```python
from build123d import *

# Parameters (mm, degrees)
SKETCH_1_R      = 20
SKETCH_1_R_2    = 1.55
EXTRUDE_1_DEPTH = 3


with BuildPart() as part:
    # 草图1 → 凸台-拉伸1 (new body)
    with BuildSketch(Plane.XY):
        with BuildLine():
            Line((-4, 6), (-4, 0))
            ThreePointArc((-4, 0), (-7.907990216, -19.039432765), (-19, -35))
            ThreePointArc((-19, -35), (-39.34333678, -74.530954843), (4.648648649, -68.108108108))
            ThreePointArc((4.648648649, -68.108108108), (13.142724005, -34.523787334), (16, 0))
            ThreePointArc((16, 0), (15.97856596, 3.000306232), (15.914268214, 6))
            Line((15.914268214, 6), (-4, 6))
        make_face()
        with Locations((-19, -60)):
            Circle(SKETCH_1_R, mode=Mode.SUBTRACT)
        with BuildLine():
            ThreePointArc((-10.997130101, -35.262294501), (-2.27235419, -21.118936487), (1.769449507, -5))
            Line((1.769449507, -5), (9.938716285, -5))
            ThreePointArc((9.938716285, -5), (8.233133382, -26.791038845), (4.205881516, -48.274512246))
            ThreePointArc((4.205881516, -48.274512246), (-2.093610856, -40.247177262), (-10.997130101, -35.262294501))
        make_face(mode=Mode.SUBTRACT)
        Circle(SKETCH_1_R_2, mode=Mode.SUBTRACT)
        with Locations((12, 0)):
            Circle(SKETCH_1_R_2, mode=Mode.SUBTRACT)
    extrude(amount=EXTRUDE_1_DEPTH)


solid = part.part
```
Verification items for the finished model (mm, model axes). A direction names the side the tool comes from. Round coordinates to 2 decimals unless told otherwise and drop trailing zeros. Write each loop counter-clockwise with the first axis right and the second up, starting at its lowest first coordinate (ties: lowest second). Pieces come first, ordered by that corner, then holes.
1. Gauge pin test, flat end, axial feed: P1, Ø1, axis at x = -14, z = 2.5, coming from the -Y side. Record the tip position at first contact, or that the pin passes through.
2. Access from +Z, -Z, +X, -X, +Y, -Y to the whole of each face (thin tool, end or side, straight path). Record for faces 1 (the flat face through (-5, -39, 3)), 2 (the flat face through (-4, 3, 1)), 3 (the flat face through (6, -5, 1)).
3. Draft check along X on faces 4 (the cylindrical face through (0.715, -1.375, 1.479)), 5 (the flat face through (-5, -39, 0)), 6 (the cylindrical face through (-7.8, -18.79, 1.48)). Enter one of: +X half, -X half, draft (parallel to the pull), parting line (faces both ways), or undercut.
4. Section check C-C on x = 0. Enter the section's corners in (y, z) (3 decimals), plus the area to 3 significant figures.
5. Section check A-A on z = 1.05. Enter the section's corners in (x, y).
6. Section check D-D on y = -28. Enter the section's corners in (x, z).
7. Scan lines: L1, parallel to Y at x = -3.5, z = 2.65; L2, parallel to X at y = -0.5, z = 2.2; L3, parallel to Y at x = -19, z = 1.5. Record each from-to range of solid material in increasing order.
8. Section check B-B on y = -43. Enter the section's corners in (x, z).
Answer:
1. P1: stops at y = -84.59
2. face 1: +Z, +X, -X, +Y, -Y
2. face 2: +Z, -Z, -X, +Y
2. face 3: +Z, -Z
3. face 4: undercut
3. face 5: draft
3. face 6: -X half
4. outline: (-76.248, 0) - (-66.245, 0) - (-66.245, 3) - (-76.248, 3) - close; (-53.755, 0) - (-42.252, 0) - (-42.252, 3) - (-53.755, 3) - close; (-14.606, 0) - (-1.55, 0) - (-1.55, 3) - (-14.606, 3) - close; (1.55, 0) - (6, 0) - (6, 3) - (1.55, 3) - close
4. area: 117 mm2
5. outline: (-19, -35) arc R25 ccw (long way) to (4.65, -68.11) arc R210 ccw to (16, 0) arc R210 ccw to (15.91, 6) - (-4, 6) - (-4, 0) arc R48.33 cw to start; hole circle Ø40 at (-19, -60); hole (-11, -35.26) arc R26 cw to (4.21, -48.27) arc R204 ccw to (9.94, -5) - (1.77, -5) arc R54.33 cw to start; hole circle Ø3.1 at (0, 0); hole circle Ø3.1 at (12, 0)
6. outline: (-12.94, 0) - (-5.77, 0) - (-5.77, 3) - (-12.94, 3) - close; (8.07, 0) - (14.12, 0) - (14.12, 3) - (8.07, 3) - close
7. L1: y = -79.62 to -72.64, -47.36 to -39.13, -23.82 to 6
7. L2: x = -4 to -1.47, 1.47 to 10.53, 13.47 to 16
7. L3: y = -85 to -80, -40 to -35
8. outline: (-37.33, 0) - (-29.54, 0) - (-29.54, 3) - (-37.33, 3) - close; (-8.46, 0) - (0.67, 0) - (0.67, 3) - (-8.46, 3) - close; (5.42, 0) - (11.55, 0) - (11.55, 3) - (5.42, 3) - close
